For this review, take the finished solid that the model builds, in its own axes (mm). Give positions to 0.01 mm unless a question says otherwise; leave off trailing zeros. Write each loop counter-clockwise with the first axis right and the second up, starting at its lowest first coordinate (ties: lowest second). Pieces come first, ordered by that corner, then holes.
1) We need section A-A on x = -18. Give the boundary of the cut face in (y, z).
2) For P1, Ø0.5, axis at x = -56, y = -0.5, coming from the +Z side, flat-tipped, find the tip position at first contact; note if it passes through.
3) We need section B-B on y = -0.25. Give the number of separate pieces and of enclosed holes in the cut face, and give its area (3 significant figures).
4) Wall thickness on line 1 along Z through (x, y) = (39, -0.2): over which ranges is the line inside the solid? List them lowest first.
from build123d import *

# Parameters (mm, degrees)
F0_W     = 10
F0_H     = 2.4
F1_DEPTH = 1.6


with BuildPart() as f1:
    # F0 (on Front) → F1 (new body)
    with BuildSketch(Plane.XZ):
        Polygon((-125.837884, 14.897037), (-125.837884, -55.102963), (-120.837884, -55.102963), (-120.837884, -55.602963), (-110.837884, -55.602963), (-110.837884, -55.102963), (-100.837884, -55.102963), (-100.837884, -55.602963), (-90.837884, -55.602963), (-90.837884, -55.102963), (-80.837884, -55.102963), (-80.837884, -55.602963), (-70.837884, -55.602963), (-70.837884, -55.102963), (-60.837884, -55.102963), (-60.837884, -55.602963), (-50.837884, -55.602963), (-50.837884, -55.102963), (-40.837884, -55.102963), (-40.837884, -55.602963), (-30.837884, -55.602963), (-30.837884, -55.102963), (-20.837884, -55.102963), (-20.837884, -55.602963), (-10.837884, -55.602963), (-10.837884, -55.102963), (-0.837884, -55.102963), (-0.837884, -55.602963), (9.162116, -55.602963), (9.162116, -55.102963), (19.162116, -55.102963), (19.162116, -55.602963), (29.162116, -55.602963), (29.162116, -55.102963), (39.162116, -55.102963), (39.162116, -55.602963), (49.162116, -55.602963), (49.162116, -55.102963), (59.162116, -55.102963), (59.162116, -55.602963), (69.162116, -55.602963), (69.162116, -55.102963), (79.162116, -55.102963), (79.162116, -55.602963), (89.162116, -55.602963), (89.162116, -55.102963), (99.162116, -55.102963), (99.162116, -55.602963), (109.162116, -55.602963), (109.162116, -55.102963), (124.662116, -55.102963), (124.662116, 14.897037), (119.162116, 14.897037), (109.162116, 14.897037), (109.162116, 14.397037), (99.162116, 14.397037), (99.162116, 14.897037), (89.162116, 14.897037), (89.162116, 14.397037), (79.162116, 14.397037), (79.162116, 14.897037), (69.162116, 14.897037), (69.162116, 14.397037), (59.162116, 14.397037), (59.162116, 14.897037), (49.162116, 14.897037), (49.162116, 14.397037), (39.162116, 14.397037), (39.162116, 14.897037), (29.162116, 14.897037), (29.162116, 14.397037), (19.162116, 14.397037), (19.162116, 14.897037), (9.162116, 14.897037), (9.162116, 14.397037), (-0.837884, 14.397037), (-0.837884, 14.897037), (-10.837884, 14.897037), (-10.837884, 14.397037), (-20.837884, 14.397037), (-20.837884, 14.897037), (-30.837884, 14.897037), (-30.837884, 14.397037), (-40.837884, 14.397037), (-40.837884, 14.897037), (-50.837884, 14.897037), (-50.837884, 14.397037), (-60.837884, 14.397037), (-60.837884, 14.897037), (-70.837884, 14.897037), (-70.837884, 14.397037), (-80.837884, 14.397037), (-80.837884, 14.897037), (-90.837884, 14.897037), (-90.837884, 14.397037), (-100.837884, 14.397037), (-100.837884, 14.897037), (-110.837884, 14.897037), (-110.837884, 14.397037), (-120.837884, 14.397037), (-120.837884, 14.897037), align=None)
        with Locations((-115.837884, -41.302963)):
            Rectangle(F0_W, F0_H, mode=Mode.SUBTRACT)
        with Locations((-95.837884, -41.302963)):
            Rectangle(F0_W, F0_H, mode=Mode.SUBTRACT)
        with Locations((-75.837884, -41.302963)):
            Rectangle(F0_W, F0_H, mode=Mode.SUBTRACT)
        with Locations((-55.837884, -41.302963)):
            Rectangle(F0_W, F0_H, mode=Mode.SUBTRACT)
        with Locations((-35.837884, -41.302963)):
            Rectangle(F0_W, F0_H, mode=Mode.SUBTRACT)
        with Locations((-15.837884, -41.302963)):
            Rectangle(F0_W, F0_H, mode=Mode.SUBTRACT)
        with Locations((4.162116, -41.302963)):
            Rectangle(F0_W, F0_H, mode=Mode.SUBTRACT)
        with Locations((24.162116, -41.302963)):
            Rectangle(F0_W, F0_H, mode=Mode.SUBTRACT)
        with Locations((44.162116, -41.302963)):
            Rectangle(F0_W, F0_H, mode=Mode.SUBTRACT)
        with Locations((64.162116, -41.302963)):
            Rectangle(F0_W, F0_H, mode=Mode.SUBTRACT)
        with Locations((84.162116, -41.302963)):
            Rectangle(F0_W, F0_H, mode=Mode.SUBTRACT)
        with Locations((104.162116, -41.302963)):
            Rectangle(F0_W, F0_H, mode=Mode.SUBTRACT)
        with Locations((-115.837884, -1.302963)):
            Rectangle(F0_W, F0_H, mode=Mode.SUBTRACT)
        with Locations((-95.837884, -1.302963)):
            Rectangle(F0_W, F0_H, mode=Mode.SUBTRACT)
        with Locations((-75.837884, -1.302963)):
            Rectangle(F0_W, F0_H, mode=Mode.SUBTRACT)
        with Locations((-55.837884, -1.302963)):
            Rectangle(F0_W, F0_H, mode=Mode.SUBTRACT)
        with Locations((-35.837884, -1.302963)):
            Rectangle(F0_W, F0_H, mode=Mode.SUBTRACT)
        with Locations((-15.837884, -1.302963)):
            Rectangle(F0_W, F0_H, mode=Mode.SUBTRACT)
        with Locations((4.162116, -1.302963)):
            Rectangle(F0_W, F0_H, mode=Mode.SUBTRACT)
        with Locations((24.162116, -1.302963)):
            Rectangle(F0_W, F0_H, mode=Mode.SUBTRACT)
        with Locations((44.162116, -1.302963)):
            Rectangle(F0_W, F0_H, mode=Mode.SUBTRACT)
        with Locations((64.162116, -1.302963)):
            Rectangle(F0_W, F0_H, mode=Mode.SUBTRACT)
        with Locations((84.162116, -1.302963)):
            Rectangle(F0_W, F0_H, mode=Mode.SUBTRACT)
        with Locations((104.162116, -1.302963)):
            Rectangle(F0_W, F0_H, mode=Mode.SUBTRACT)
    extrude(amount=F1_DEPTH)


solid = f1.part
Results list:
1. outline: (-1.6, -55.6) - (0, -55.6) - (0, -42.5) - (-1.6, -42.5) - close; (-1.6, -40.1) - (0, -40.1) - (0, -2.5) - (-1.6, -2.5) - close; (-1.6, -0.1) - (0, -0.1) - (0, 14.4) - (-1.6, 14.4) - close
2. P1: stops at z = 14.4
3. separate pieces: 1
3. enclosed holes: 24
3. area: 17,000 mm2
4. line 1: z = -55.1 to 14.9
